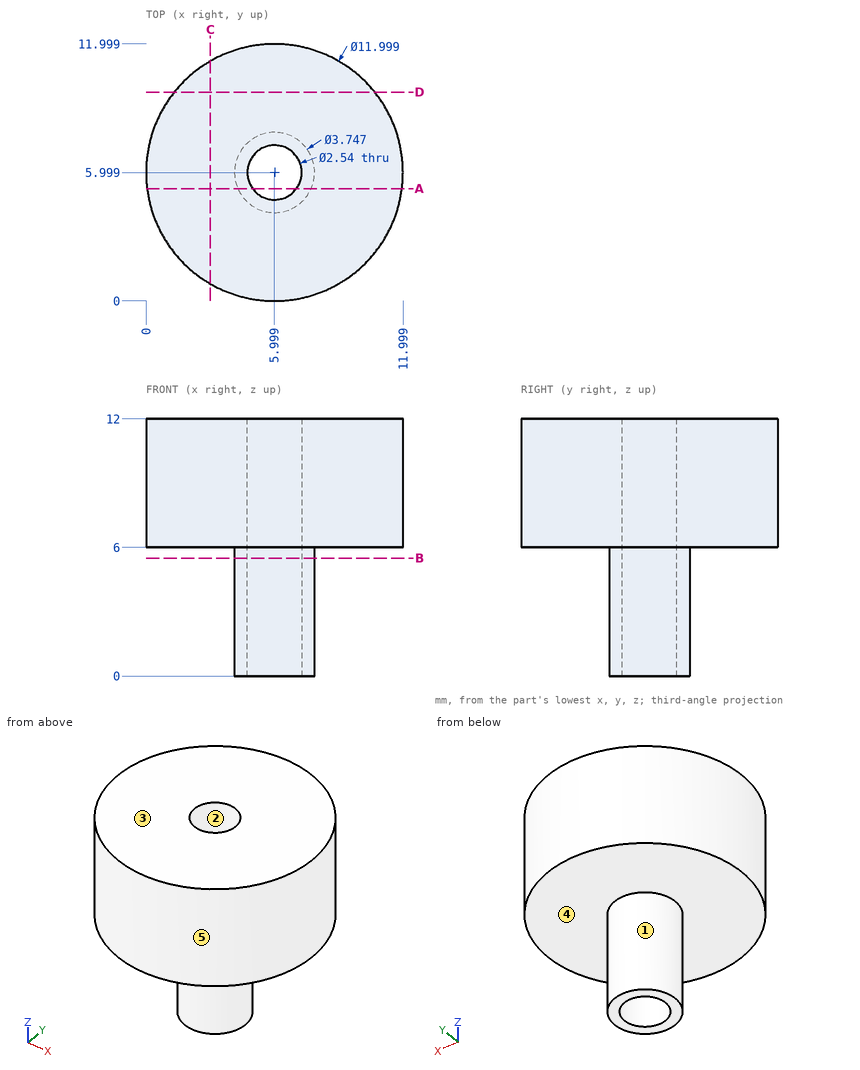
Study the drawing (mm; zero at the part's minimum x, y, z) and answer. A direction names the side the tool comes from. Coordinates: 2 decimals unless noted, no trailing zeros. Loops run counter-clockwise (first coordinate to the right, second up) from the corner with the lowest first, then second, coordinate; pieces in that order, holes last. Notation, with made-up numbers: M 34.5,-16 L 66.5,-16 A15 ccw 66.5,5 Z; hole C 37.5,36 d4. An arc over 180 degrees is marked long. Answer in a Markdown table with one row per item. Add a question column.
1. A tool of negligible diameter and unlimited length cuts with its end or side. For the marked faces 4 and 5, from which of +Z, -Z, +X, -X, +Y, -Y can it reach the whole face along a straight path? Write none if from no direction.
2. The mould has two halves that part along X. Classify the marked faces 1, 2 and 3: pulls with the +X half, pulls with the -X half, needs draft (parallel to the pull), parting line crosses it, or undercut.
3. Find section A-A, the plane y = 5.25. Write down the section's boundary in (x, z) (1 decimal).
4. Find section B-B, the plane z = 5.5. Write down the section's boundary in (x, y).
5. Flat-ended cylindrical pins translate along their axes: P1, Ø6, axis at x = 2.5, z = 4, coming from the +Y side (1 decimal); P2, Ø2, axis at x = 6, y = 6, coming from the +Z side; P3, Ø3, axis at y = 3.5, z = 9, coming from the +X side (1 decimal); P4, Ø4, axis at x = 3, y = 8.5, coming from the -Z side. Find the tip coordinate at first contact, or state that the pin passes through.
6. Find section D-D, the plane y = 9.75. Write down the section's boundary in (x, z).
7. Consider L1, parallel to Z at x = 6.5, y = 0.5; L2, parallel to Y at x = 5.75, z = 1.5 (1 decimal); L3, parallel to Y at x = 7, z = 8.75 (1 decimal). Determine where each line is inside the solid, lowest interval first.
8. Find section C-C, the plane x = 3. Write down the section's boundary in (y, z) (1 decimal).
Reported:
| question | item | result |
|---|---|---|
| 1 | face 4 | -Z |
| 1 | face 5 | +Z, -Z |
| 2 | face 1 | parting line crosses it |
| 2 | face 2 | undercut |
| 2 | face 3 | needs draft |
| 3 | outline | M 0,6 L 4.3,6 L 4.3,0 L 5,0 L 5,12 L 0,12 Z; M 7,0 L 7.7,0 L 7.7,6 L 12,6 L 12,12 L 7,12 Z |
| 4 | outline | C 6,6 d3.75; hole C 6,6 d2.54 |
| 5 | P1 | stops at y = 11.9 |
| 5 | P2 | passes through |
| 5 | P3 | stops at x = 11.9 |
| 5 | P4 | stops at z = 6 |
| 6 | outline | M 1.32,6 L 10.68,6 L 10.68,12 L 1.32,12 Z |
| 7 | L1 | z = 6 to 12 |
| 7 | L2 | y = 4.1 to 4.8, 7.2 to 7.9 |
| 7 | L3 | y = 0.1 to 5.2, 6.8 to 11.9 |
| 8 | outline | M 0.8,6 L 11.2,6 L 11.2,12 L 0.8,12 Z |
